Can you work these out from the model? Positions are in its coordinate system, mm. A direction names the side the tool comes from. Coordinates: 2 decimals unless noted, no trailing zeros. Order: outer loops, then holes, each group sorted by start corner. A loop starts at its lowest first (then second) coordinate and runs counter-clockwise, first axis right, second up. Notation, with made-up numbers: (67, 80) -> (87, 80) arc R24 cw to (87, 96) -> close; hole circle Ø8 at (44, 70.25). An arc over 180 degrees is marked (long way). Answer as CSV lines item,"result".
Autodesk Inventor part; units mm, degrees
ref_plane "作業平面5" through (0, -6, 90) normal (0, -1, 0) x (1, 0, 0)
ref_plane "YZ Plane" through (0, 0, 0) normal (1, 0, 0) x (0, 1, 0)
ref_plane "XZ Plane" through (0, 0, 0) normal (0, 1, 0) x (-1, 0, 0)
sketch "スケッチ1" plane through (0, 0, 0) normal (0, 0, 1) x (1, 0, 0)
  circle A0 centre (0, 0) radius 5
  dimension "d0" = 10
extrude "押し出し1" add sketch "スケッチ1" along normal blind 35
thread "ねじ1"
sketch "スケッチ2" plane through (0, 0, 35) normal (0, 0, 1) x (1, 0, 0)
  circle A0 centre (0, 0) radius 6
  dimension "d5" = 12
extrude "押し出し2" add sketch "スケッチ2" along normal blind 55
sketch "スケッチ6" plane through (0, 0, 90) normal (0, 0, 1) x (1, 0, 0)
  line L0 (0, 0) -> (0, -6) construction
  circle A0 centre (0, 0) radius 6
ref_plane "作業平面5" through (0, -6, 90) normal (0, -1, 0) x (1, 0, 0)
sketch "スケッチ8" plane through (0, -6, 90) normal (0, -1, 0) x (1, 0, 0)
  line L0 (6, 0) -> (-6, 0)
  line L1 (-2, 0) -> (2, 0)
  line L2 (-2, 0) -> (2, 0)
  line L3 (2, 0) -> (2, -48)
  line L4 (-2, -48) -> (-2, 0)
  arc A0 (-2, -48) -> (2, -48) centre (0, -48) ccw
  point P0 (0, -90)
  point P1 (0, 0)
  dimension "d11" = 2
  dimension "d17" = 48
  dimension "d29" = 2
extrude "押し出し3" cut sketch "スケッチ8" against normal blind 2.157
sketch "スケッチ9" plane through (0, 0, 90) normal (0, 0, 1) x (1, 0, 0)
  point P0 (0, 0)
  point P1 (0, 0)
hole "穴1" at (0, 0, 90) direction (0, 0, -1) diameter 5 depth 8 tip angle 118
thread "ねじ2"
thread "ねじ3"
properties part number "正しい"
Q1. Imagine slicing it at A-A (y = 3.5). List the corners of the cut face in (x, z) for me, and give its area (3 significant figures).
Solution:
outline,"(-4.87, 35) -> (-3.57, 35) -> (-3.57, 0) -> (3.57, 0) -> (3.57, 35) -> (4.87, 35) -> (4.87, 90) -> (-4.87, 90) -> close"
area,"786 mm2"
Q2. If I drill on line 1 (Y direction, x = 0, z = 84.5); line 2 (X direction, y = 0, z = 88); line 3 (X direction, y = -4, z = 55.5), over which ranges is the centre line in solid material (lowest first)?
Solution:
line 1,"-3.84 to -2.5, 2.5 to 6"
line 2,"-6 to -2.5, 2.5 to 6"
line 3,"-4.47 to -2, 2 to 4.47"
Q3. Imagine slicing it at C-C (z = 24). List the corners of the cut face in (x, y) for me.
Solution:
outline,"circle Ø10 at (0, 0)"
Q4. We'd pull the mould along X, two halves only. Please class faces 4 (the flat face through (-4, 4, 35)), 5 (the cylindrical face through (-1.301, 5.857, 62.115)), 6 (the cylindrical face through (2.44, 0.54, 85.94)): pulls with the +X half, pulls with the -X half, needs draft (parallel to the pull), parting line crosses it, or undercut.
Solution:
face 4,"needs draft"
face 5,"parting line crosses it"
face 6,"undercut"
Q5. For P1, Ø2, axis at y = -5, z = 62.5, coming from the -X side; P2, Ø0.5, axis at y = -4.5, z = 59.5, coming from the +X side; P3, Ø4, axis at x = 0, z = 15, coming from the +Y side, each with a flat end and sliding along its axis, tell me the tip position at first contact or that it passes through.
Solution:
P1,"x = -4.47"
P2,"x = 4.24"
P3,"y = 5"
Q6. Imagine slicing it at D-D (z = 37.5). List the corners of the cut face in (x, y) for me.
Solution:
outline,"circle Ø12 at (0, 0)"
Q7. Imagine slicing it at B-B (z = 48.5). List the corners of the cut face in (x, y) for me, and give its area (3 significant figures).
Solution:
outline,"(-2, -5.66) -> (-2, -3.84) -> (2, -3.84) -> (2, -5.66) arc R6 ccw (long way) to start"
area,"105 mm2"
Q8. Which directions (+Z, -Z, +X, -X, +Y, -Y) give clear straight access to the entire face, cutting with the end or side of a thin tool? Please do faces 1 (the cylindrical face through (0, -5, 40)), 2 (the flat face through (0, 3, 90)), 3 (the cylindrical face through (-1.08, 4.88, 17.26)).
Solution:
face 1,"+Z, -Y"
face 2,"+Z, +X, -X, +Y, -Y"
face 3,"-Z"
